Answer from the drawing. Dimensions are ordinates in mm from the lowest x, y and z of the part. Coordinates: 2 decimals unless noted, no trailing zeros. Write each loop counter-clockwise with the first axis right and the second up, starting at its lowest first coordinate (ties: lowest second). Pieces come first, ordered by that corner, then holes.
1) Find the intervals of material crossed by line 1 (Y direction, x = 92, z = 0.9); line 2 (Y direction, x = 10, z = 0.6); line 3 (X direction, y = 9, z = 0.5), in increasing order.
2) The part is cut by section C-C (x = 10). Determine the outline of the cut face in (y, z).
3) The part is cut by section A-A (x = 48). Determine the outline of the cut face in (y, z).
4) The part is cut by section B-B (z = 1.35). Determine the outline of the cut face in (x, y), then the cut area to 3 significant figures.
5) This flat-tipped pin is pushed along its axis until it touches: pin 1 Ø4.5 at (x, y) = (130, 10) entering from -Z. Where does it stop, or does it pass through?
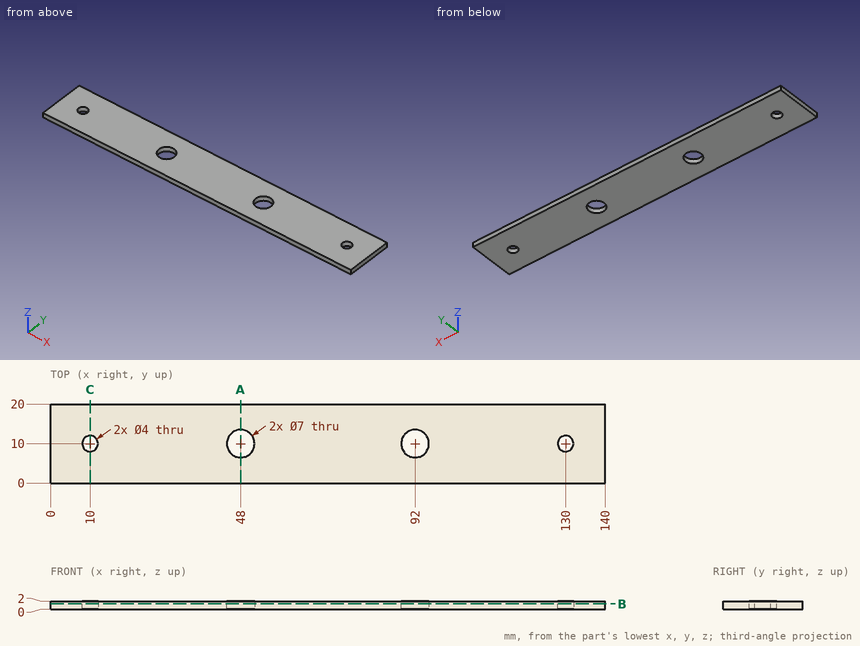
Reported:
1. line 1: y = 0 to 6.5, 13.5 to 20
1. line 2: y = 0 to 8, 12 to 20
1. line 3: x = 0 to 8.27, 11.73 to 44.65, 51.35 to 88.65, 95.35 to 128.27, 131.73 to 140
2. outline: (0, 0) - (8, 0) - (8, 2) - (0, 2) - close; (12, 0) - (20, 0) - (20, 2) - (12, 2) - close
3. outline: (0, 0) - (6.5, 0) - (6.5, 2) - (0, 2) - close; (13.5, 0) - (20, 0) - (20, 2) - (13.5, 2) - close
4. outline: (0, 0) - (140, 0) - (140, 20) - (0, 20) - close; hole circle Ø4 at (10, 10); hole circle Ø7 at (48, 10); hole circle Ø7 at (92, 10); hole circle Ø4 at (130, 10)
4. area: 2,700 mm2
5. pin 1: stops at z = 0
